Input: part model. Units: mm. Frame: model coordinates. Face numbers are marked on the shaded views. A direction names the side the tool comes from. Round coordinates to 2 decimals unless told otherwise and drop trailing zeros. Loops run counter-clockwise (first coordinate to the right, second up) from the corner with the lowest first, then second, coordinate; pieces in that order, holes last. Notation, with made-up numbers: (-23, 69) - (24, 69) arc R25 cw to (24, 104) - close; hole circle Ø11 at (65.25, 63). An arc over 180 degrees is marked (long way). Use CSV: the item, a comma, the result in double quotes. Start each with the question number.
1. Cut plane D-D (z = 7.5). Return loops of the section in (x, y), and give its area (3 significant figures).
2. Pull-direction query (Z, two-part tool) for the marked faces 4, 5 and 6; classes: +Z half, -Z half, draft (parallel to the pull), parting line (faces both ways), or undercut.
3. Pin query (flat end, axial travel): P1, Ø5, axis at x = 0, y = 0, coming from the -Z side; P2, Ø1.5, axis at y = -0.5, z = 6, coming from the +X side; P3, Ø0.9, axis at y = 0.5, z = 7, coming from the -X side; P4, Ø3.5, axis at x = 0.5, z = 6, coming from the +Y side. Return the tip coordinate at first contact, or that it passes through.
4. Cut plane B-B (z = 22). Return loops of the section in (x, y).
5. Access query for the marked faces 1, 2 and 3. Directions: +Z, -Z, +X, -X, +Y, -Y. A direction counts if a zero-diameter tool reaches every point of the face in a straight line with its end or side. Return the directions, or none.
6. Material intervals for probe 1 along Y at (x, z) = (0, 3.35); probe 2 along Y at (x, z) = (-1.25, 29); probe 3 along X at (y, z) = (0, 3.75), sorted ascending. Write a range as from..to.
```python
from build123d import *

# Parameters (mm, degrees)
CROQUIS1_R              = 2.5
CROQUIS1_R_2            = 1.8
SALIENTE_EXTRUIR1_DEPTH = 7
SALIENTE_EXTRUIR2_REACH = 9.842
CROQUIS3_R              = 3.5
CROQUIS3_R_2            = 1.6
CROQUIS4_W              = 10
CROQUIS4_H              = 10
SALIENTE_EXTRUIR3_DEPTH = 1
REDONDEO2_R             = 1.5
CROQUIS7_W              = 3.5
CROQUIS7_H              = 3.5
CORTAR_EXTRUIR1_DEPTH   = 3
SALIENTE_EXTRUIR4_DEPTH = 22
CROQUIS9_W              = 10
CROQUIS9_H              = 10
SALIENTE_EXTRUIR5_DEPTH = 1.5


with BuildPart() as part:
    # Croquis1 → Saliente-Extruir1 (new body)
    with BuildSketch(Plane.XY):
        Circle(CROQUIS1_R)
        Circle(CROQUIS1_R_2, mode=Mode.SUBTRACT)
    extrude(amount=SALIENTE_EXTRUIR1_DEPTH)

    # Saliente-Extruir2: up to this plane
    saliente_extruir2_end = Plane(origin=(0, 1.223696204, 3.362077689), z_dir=(0, -0.34202014332567576, -0.9396926207859059))
    # Croquis3 → Saliente-Extruir2 (add, up to the surface)
    with BuildSketch(Plane.XY.offset(7), mode=Mode.PRIVATE) as saliente_extruir2_sk1:
        Circle(CROQUIS3_R)
        Circle(CROQUIS3_R_2, mode=Mode.SUBTRACT)
    saliente_extruir2_tool1 = split(extrude(saliente_extruir2_sk1.sketch, amount=-SALIENTE_EXTRUIR2_REACH, mode=Mode.PRIVATE), bisect_by=saliente_extruir2_end, keep=Keep.BOTH, mode=Mode.PRIVATE)
    add(saliente_extruir2_tool1.solids().sort_by_distance((-3.401005, 0, 7))[0])

    # Croquis4 → Saliente-Extruir3 (add)
    with BuildSketch(Plane.XY.offset(7)):
        Rectangle(CROQUIS4_W, CROQUIS4_H)
    extrude(amount=SALIENTE_EXTRUIR3_DEPTH)

    # Redondeo2
    # the kernel refuses this fillet: 1.5 mm, written as the material it takes off along each edge
    with BuildSketch(Plane(origin=(-5, -8.535533906, 7), x_dir=(0, 0, 1), z_dir=(0, 1, 0)), Plane(origin=(8.535533906, -5, 7), x_dir=(0, 0, 1), z_dir=(-1, 0, 0)), Plane(origin=(5, 8.535533906, 7), x_dir=(0, 0, 1), z_dir=(0, -1, 0))) as redondeo2_piece_1:
        with BuildLine():
            CenterArc((1.5, 1.414213562), REDONDEO2_R, 180, 70.528779366)
            Line((0, 1.414213562), (-0.03, 1.414213562))
            Line((-0.03, 1.414213562), (-0.03, 0))
            Line((-0.03, 0), (0, -0.03))
            ThreePointArc((0, -0.03), (0.5, -0.03), (0.99, -0.028284271))
            Line((0.99, -0.028284271), (1, 0))
        make_face()
    extrude(amount=17.071067812, mode=Mode.SUBTRACT)
    with BuildSketch(Plane(origin=(-8.535533906, 5, 7), x_dir=(0, -1, 0), z_dir=(1, 0, 0))) as redondeo2_piece_2:
        with BuildLine():
            CenterArc((1.414213562, -1.5), REDONDEO2_R, 90, 70.528779366)
            Line((0, -1), (-0.028284271, -0.99))
            ThreePointArc((-0.028284271, -0.99), (-0.03, -0.5), (-0.03, 0))
            Line((-0.03, 0), (0, 0.03))
            Line((0, 0.03), (1.414213562, 0.03))
            Line((1.414213562, 0.03), (1.414213562, 0))
        make_face()
    extrude(amount=17.071067812, mode=Mode.SUBTRACT)

    # Croquis7 → Cortar-Extruir1 (cut)
    with BuildSketch(Plane.XY.offset(8)):
        Rectangle(CROQUIS7_W, CROQUIS7_H)
    extrude(amount=-CORTAR_EXTRUIR1_DEPTH, mode=Mode.SUBTRACT)

    # Croquis8 → Saliente-Extruir4 (add)
    with BuildSketch(Plane.XY.offset(8)):
        Polygon((3.75, 5), (-5, 5), (-5, -5), (3.75, -5), (5, -5), (5, -3.75), (3.75, -3.75), (-3.75, -3.75), (-3.75, 3.75), (3.75, 3.75), (5, 3.75), (5, 5), align=None)
    extrude(amount=SALIENTE_EXTRUIR4_DEPTH)

    # Croquis9 → Saliente-Extruir5 (add)
    with BuildSketch(Plane.XY.offset(30)):
        Rectangle(CROQUIS9_W, CROQUIS9_H)
    extrude(amount=SALIENTE_EXTRUIR5_DEPTH)


solid = part.part
```
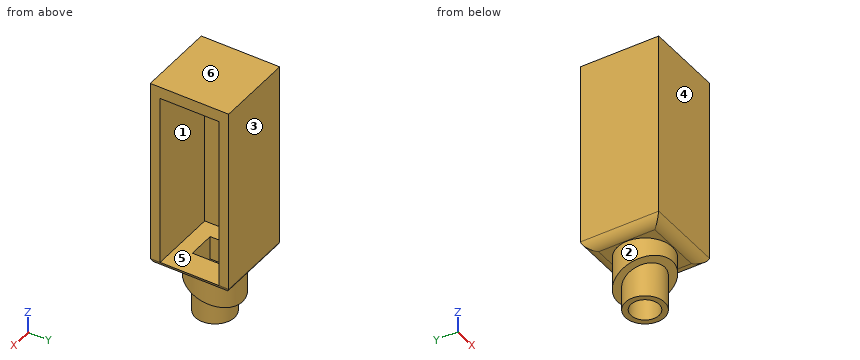
Established:
1,outline,"(-4.7, -4.7) - (4.7, -4.7) - (4.7, 4.7) - (-4.7, 4.7) - close; hole (-1.75, -1.75) - (1.75, -1.75) - (1.75, 1.75) - (-1.75, 1.75) - close"
1,area,"76.3 mm2"
2,face 4,"draft"
2,face 5,"undercut"
2,face 6,"+Z half"
3,P1,"stops at z = 0"
3,P2,"stops at x = 3.5"
3,P3,"stops at x = -4.66"
3,P4,"stops at y = 4.88"
4,outline,"(-5, -5) - (5, -5) - (5, -3.75) - (-3.75, -3.75) - (-3.75, 3.75) - (5, 3.75) - (5, 5) - (-5, 5) - close"
5,face 1,"+X"
5,face 2,"-Z"
5,face 3,"+Z, -Z, +X, -X, +Y"
6,probe 1,"y = -2.5..-1.8, 1.6..3.5"
6,probe 2,"y = -5..-3.75, 3.75..5"
6,probe 3,"x = -2.5..-1.8, 1.8..2.5"
